Model file for the job. Use its own axes, mm. Round coordinates to 2 decimals unless told otherwise and drop trailing zeros. Order: outer loops, then holes, each group sorted by start corner. A loop starts at its lowest first (then second) coordinate and runs counter-clockwise, first axis right, second up. Notation, with made-up numbers: (55, 51.5) - (78, 51.5) arc R25 ccw to (78, 71.5) - close; hole circle Ø5 at (26, 65.5). An arc over 180 degrees is marked (long way). Write item = value, one per line.
```python
from build123d import *

# Parameters (mm, degrees)
ESQUISSE1_R             = 3
BOSS_EXTRU_1_DEPTH      = 10
ENL_V_START             = -10
ESQUISSE2_R             = 3
ENL_V_MAT_EXTRU_1_DEPTH = 10


with BuildPart() as part:
    # Esquisse1 → Boss.-Extru.1 (new body)
    with BuildSketch(Plane.XY):
        with BuildLine():
            Line((-122.628083491, -8.225806452), (387.371916509, -8.225806452))
            ThreePointArc((387.371916509, -8.225806452), (397.371916509, -18.225806452), (387.371916509, -28.225806452))
            Line((387.371916509, -28.225806452), (-122.628083491, -28.225806452))
            ThreePointArc((-122.628083491, -28.225806452), (-132.628083491, -18.225806452), (-122.628083491, -8.225806452))
        make_face()
        with Locations((-117.628083491, -18.225806452)):
            Circle(ESQUISSE1_R, mode=Mode.SUBTRACT)
        with Locations((382.371916509, -18.225806452)):
            Circle(ESQUISSE1_R, mode=Mode.SUBTRACT)
    extrude(amount=BOSS_EXTRU_1_DEPTH)

    # Esquisse2 → Enlèv. mat.-Extru.1 (cut)
    with BuildSketch(Plane.XY.offset(10).offset(ENL_V_START)):
        with Locations((132.370892359, -17.510213181)):
            Circle(ESQUISSE2_R)
        with Locations((-117.628083491, -18.225806452)):
            Circle(ESQUISSE2_R)
    extrude(amount=ENL_V_MAT_EXTRU_1_DEPTH, mode=Mode.SUBTRACT)


solid = part.part
```
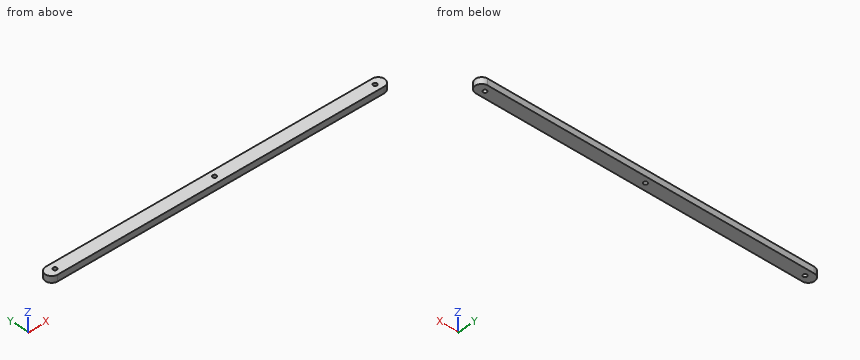
1) Cut at A-A (z = 5.25). Write the cut outline in (x, y), and give its area (3 significant figures).
Conclusion:
outline = (-122.63, -28.23) - (387.37, -28.23) arc R10 ccw to (387.37, -8.23) - (-122.63, -8.23) arc R10 ccw to start; hole circle Ø6 at (-117.63, -18.23); hole circle Ø6 at (132.37, -17.51); hole circle Ø6 at (382.37, -18.23)
area = 10,400 mm^2
2) Wall check: line 1 along X through (y, z) = (-14.75, 5.75); line 2 along X through (y, z) = (-24.75, 1); line 3 along X through (y, z) = (-13.5, 5.5). Give the ranges that are in metal, low to high.
Conclusion:
line_1 = -132 to 131.2, 133.55 to 396.75
line_2 = -130.21 to 394.95
line_3 = -131.44 to 396.18
3) Flat gauge pins, fed straight in: pin 1 Ø3 at (y, z) = (-15, 4) entering from +X; pin 2 Ø5.5 at (x, y) = (132.37, -17.51) entering from +Z; pin 3 Ø3 at (y, z) = (-24, 7) entering from -X; pin 4 Ø1 at (y, z) = (-15, 6.5) entering from +X. Where does each tip first touch, or does it go through?
Conclusion:
pin_1 = 397.22
pin_2 = through
pin_3 = -131.67
pin_4 = 396.99
